Input: part model. Units: mm. Frame: model coordinates. Face numbers are marked on the shaded views. Give positions to 0.01 mm unless a question says otherwise; leave off trailing zeros. Order: outer loops, then holes, each group sorted by start corner. A loop starts at its lowest first (then second) coordinate and runs counter-clockwise, first axis right, second up. Notation, with made-up numbers: (28.25, -29.75) - (48.25, -29.75) arc R17 ccw to (48.25, -16.75) - close; hole circle Ø1 at (55.25, 21.5). An arc over 180 degrees is marked (long way). Use a Markdown table: item, result.
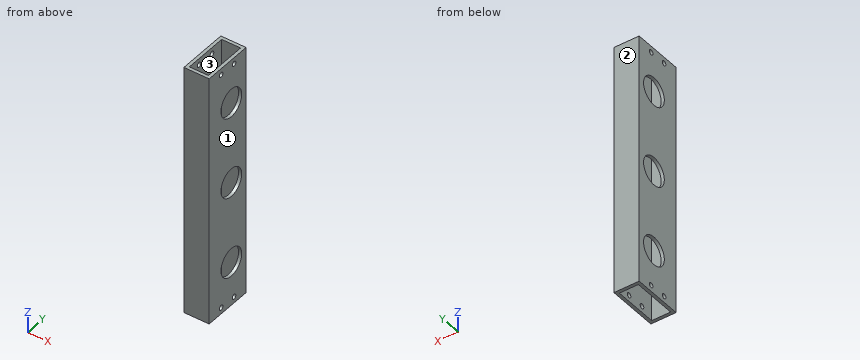
from build123d import *

# Parameters (mm, degrees)
SKETCH1_W              = 254
SKETCH1_H              = 50.8
BOSS_EXTRUDE1_DEPTH    = 25.4
SHELL1_T               = -3.175
SKETCH2_R              = 14.2875
CUT_EXTRUDE1_DEPTH     = 132.982271537
F_10_CLEARANCE_HOLE1_D = 4.9784


with BuildPart() as part:
    # Sketch1 → Boss-Extrude1 (new body)
    with BuildSketch(Plane(origin=(0, 0, 0), x_dir=(0, 0, -1), z_dir=(1, 0, 0))):
        Rectangle(SKETCH1_W, SKETCH1_H)
    extrude(amount=BOSS_EXTRUDE1_DEPTH)

    # Shell1
    shell1_openings = [part.faces().sort_by_distance(p)[0] for p in [
        (12.7, 0, 127),
        (12.7, 0, -127),
    ]]
    offset(amount=SHELL1_T, openings=shell1_openings, kind=Kind.INTERSECTION)

    # Sketch2 → Cut-Extrude1 (cut, through all)
    with BuildSketch(Plane(origin=(25.4, 0, 0), x_dir=(0, 0, -1), z_dir=(1, 0, 0))):
        with Locations((0, 5.08)):
            Circle(SKETCH2_R)
        with Locations((-82.55, 5.08)):
            Circle(SKETCH2_R)
        with Locations((82.55, 5.08)):
            Circle(SKETCH2_R)
    extrude(amount=-CUT_EXTRUDE1_DEPTH, mode=Mode.SUBTRACT)

    # #10 Clearance Hole1 (through all)
    with Locations(Plane(origin=(25.4, 0, 0), x_dir=(0, 0, -1), z_dir=(1, 0, 0))):
        with Locations((-120.65, 8.89), (-120.65, -8.89)):
            f_10_clearance_hole1 = Hole(F_10_CLEARANCE_HOLE1_D / 2)

    # Mirror1: #10 Clearance Hole1 across plane
    add(f_10_clearance_hole1.mirror(Plane.XY), mode=Mode.SUBTRACT)


solid = part.part
1. Section query B-B (x = 6.75). Return loops of the section in (y, z) (3 decimals), then the cut area to 3 significant figures.
Response:
| item | result |
|---|---|
| outline | (-25.4, -127) - (-22.225, -127) - (-22.225, 127) - (-25.4, 127) - close; (22.225, -127) - (25.4, -127) - (25.4, 127) - (22.225, 127) - close |
| area | 1,610 mm^2 |
2. Section query D-D (y = -3). State how many separate pieces and enclosed holes the cut face has, then the cut area to 3 significant figures.
Response:
| item | result |
|---|---|
| separate pieces | 8 |
| enclosed holes | 0 |
| area | 1,160 mm^2 |
3. Section query C-C (z = 0). Return loops of the section in (x, y) (1 decimal).
Response:
| item | result |
|---|---|
| outline | (0, -25.4) - (25.4, -25.4) - (25.4, -9.2) - (22.2, -9.2) - (22.2, -22.2) - (3.2, -22.2) - (3.2, -9.2) - (0, -9.2) - close; (0, 19.4) - (3.2, 19.4) - (3.2, 22.2) - (22.2, 22.2) - (22.2, 19.4) - (25.4, 19.4) - (25.4, 25.4) - (0, 25.4) - close |
4. Mould query, pull axis X, two halves, no side actions, for the marked faces 1, 2 and 3. Classes: pulls with the +X half, pulls with the -X half, needs draft (parallel to the pull), parting line crosses it, or undercut.
Response:
| item | result |
|---|---|
| face 1 | pulls with the +X half |
| face 2 | needs draft |
| face 3 | undercut |
5. Section query A-A (z = -120.65). Return loops of the section in (x, y) (3 decimals), then the cut area to 3 significant figures.
Response:
| item | result |
|---|---|
| outline | (0, -25.4) - (25.4, -25.4) - (25.4, -11.379) - (22.225, -11.379) - (22.225, -22.225) - (3.175, -22.225) - (3.175, -11.379) - (0, -11.379) - close; (0, -6.401) - (3.175, -6.401) - (3.175, 6.401) - (0, 6.401) - close; (0, 11.379) - (3.175, 11.379) - (3.175, 22.225) - (22.225, 22.225) - (22.225, 11.379) - (25.4, 11.379) - (25.4, 25.4) - (0, 25.4) - close; (22.225, -6.401) - (25.4, -6.401) - (25.4, 6.401) - (22.225, 6.401) - close |
| area | 380 mm^2 |
6. Material intervals for line 1 along Y through (x, z) = (1.15, -120.65); line 2 along X through (y, z) = (-12.5, 19.5) (3 decimals); line 3 along Y through (x, z) = (11.25, 112.5) (3 decimals), sorted ascending.
Response:
| item | result |
|---|---|
| line 1 | y = -25.4 to -11.38, -6.4 to 6.4, 11.38 to 25.4 |
| line 2 | x = 0 to 3.175, 22.225 to 25.4 |
| line 3 | y = -25.4 to -22.225, 22.225 to 25.4 |
